Build history of the part. All positions in model axes, mm. Face numbers are marked on the shaded views. A direction names the side the tool comes from. Round coordinates to 2 decimals unless told otherwise and drop trailing zeros. Write each loop counter-clockwise with the first axis right and the second up, starting at its lowest first coordinate (ties: lowest second). Pieces come first, ordered by that corner, then holes. Notation, with made-up numbers: (69, -6) -> (79, -6) arc R36 cw to (79, 33) -> close; hole circle Ø2 at (-33, -39.5). An arc over 180 degrees is marked (long way). Answer in a Markdown table with one row per item.
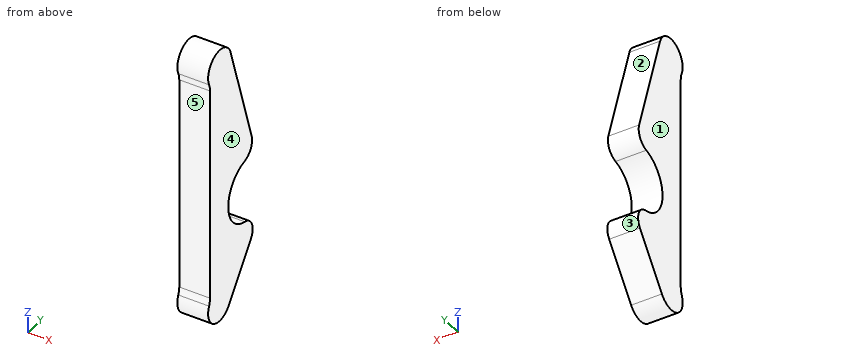
```python
from build123d import *

# Parameters (mm, degrees)
BOSS_EXTRUDE1_DEPTH = 10


with BuildPart() as part:
    # Sketch1 → Boss-Extrude1 (new body)
    with BuildSketch(Plane(origin=(0, 0, 0), x_dir=(0, 0, -1), z_dir=(1, 0, 0))):
        with BuildLine():
            Line((-45.204168477, -20), (25.204168477, -20))
            ThreePointArc((25.204168477, -20), (26.428913348, -20.126329938), (27.602084238, -20.5))
            ThreePointArc((27.602084238, -20.5), (35.194165826, -18.003438259), (33.570567469, -10.178065953))
            Line((33.570567469, -10.178065953), (18.135704254, 1.251211168))
            ThreePointArc((18.135704254, 1.251211168), (13.371146439, 1.87224401), (10.33172294, -1.849126403))
            ThreePointArc((10.33172294, -1.849126403), (0.10386055, -10.495379), (-10.293105897, -2.053226328))
            ThreePointArc((-10.293105897, -2.053226328), (-12.616026385, 1.228698191), (-16.609464476, 1.697142804))
            Line((-16.609464476, 1.697142804), (-51.78615696, -9.272029739))
            ThreePointArc((-51.78615696, -9.272029739), (-55.622311914, -17.095139314), (-47.602084238, -20.5))
            ThreePointArc((-47.602084238, -20.5), (-46.428913348, -20.126329938), (-45.204168477, -20))
        make_face()
    extrude(amount=BOSS_EXTRUDE1_DEPTH)


solid = part.part
```
Q1. Two-plate mould, pull along Z, no slides. Class the marked faces 1, 2 and 3: released by +Z, released by -Z, zero draft, split by the parting line, or undercut.
A:
| item | result |
|---|---|
| face 1 | zero draft |
| face 2 | released by +Z |
| face 3 | undercut |
Q2. Which spindle directions (+Z, -Z, +X, -X, +Y, -Y) get a long thin tool onto all of the face, cutting with end or side? Do the marked faces 4 and 5. Say none if no direction does.
A:
| item | result |
|---|---|
| face 4 | +Z, -Z, +X, +Y, -Y |
| face 5 | +X, -X, -Y |
Q3. Drop flat-ended pins along their axis: P1, Ø4, axis at x = 2, z = -11, coming from the -Y side; P2, Ø3, axis at x = 2.5, y = -3, coming from the -Z side. Give the stop position or say it passes through.
A:
| item | result |
|---|---|
| P1 | y = -20 |
| P2 | z = -25.9 |
Q4. Saw through at D-D on y = -19. Write the cut outline in (x, z), plus the area to 3 significant figures.
A:
| item | result |
|---|---|
| outline | (0, -34.47) -> (10, -34.47) -> (10, 54.47) -> (0, 54.47) -> close |
| area | 889 mm² |
Q5. Saw through at A-A on x = 5.5. Write the cut outline in (y, z), plus the area to 3 significant figures.
A:
| item | result |
|---|---|
| outline | (-20.5, -27.6) arc R6 ccw to (-10.18, -33.57) -> (1.25, -18.14) arc R4.94 ccw to (-1.85, -10.33) arc R10.5 cw to (-2.05, 10.29) arc R4.94 ccw to (1.7, 16.61) -> (-9.27, 51.79) arc R6 ccw (long way) to (-20.5, 47.6) arc R6 cw to (-20, 45.2) -> (-20, -25.2) arc R6 cw to start |
| area | 1,410 mm² |
Q6. Wall check: line 1 (Y direction, x = 4, z = 15.5); line 2 (Y direction, x = 0.5, z = 41); line 3 (Z direction, x = 3.5, y = -12.5). Give the ranges that are in metal, low to high. Write a range as [from, to].
A:
| item | result |
|---|---|
| line 1 | [-20, 1.91] |
| line 2 | [-20, -5.91] |
| line 3 | [-35.45, 55.45] |
Q7. Saw through at B-B on y = -3.5. Write the cut outline in (x, z), plus the area to 3 significant figures.
A:
| item | result |
|---|---|
| outline | (0, -24.55) -> (10, -24.55) -> (10, -9.9) -> (0, -9.9) -> close; (0, 9.9) -> (10, 9.9) -> (10, 33.28) -> (0, 33.28) -> close |
| area | 380 mm² |
Q8. Saw through at C-C on z = 33. Write the cut outline in (x, y), plus the area to 3 significant figures.
A:
| item | result |
|---|---|
| outline | (0, -20) -> (10, -20) -> (10, -3.41) -> (0, -3.41) -> close |
| area | 166 mm² |
